Geometry: final body of the model. Coordinates: model frame, mm. A direction names the side the tool comes from. Round coordinates to 2 decimals unless told otherwise and drop trailing zeros. Order: outer loops, then holes, each group sorted by start corner. A loop starts at its lowest first (then second) coordinate and runs counter-clockwise, first axis right, second up. Notation, with made-up numbers: M -35.5,-17.5 L -30.5,-17.5 A9 ccw -30.5,-5.5 Z; hole C 47.5,59 d8. An arc over 180 degrees is marked long. Return JSON: item names as keys, results as strings. Group by question number.
Q1. Contact query for flat-ended pins moving along their axis: pin 1 (7.5 mm diameter, centred on y = -45.5, z = 6, fed in from -X); pin 2 (3.5 mm diameter, centred on x = -15, z = -2, fed in from -Y). Output: stop coordinate, or through.
Q2. Cut plane B-B on y = -4. Output: boundary loops of the cut face in (x, z), and give its area (3 significant figures).
Q3. Mould query, pull axis X, two halves, no side actions, for faces 6 (the face through (0.84, -28.9, 29.99)), 7 (the face through (-14, -1, 0)), 8 (the face through (7, 0, 0)). Classes: released by +X, released by -X, zero draft, split by the parting line, or undercut.
Q4. Ray query, probe 1 along Y at (x, z) = (0, 26); probe 2 along Z at (x, y) = (0.5, -34); probe 3 along Y at (x, z) = (-5, 21.5). Return the intervals inside material, ascending.
Q5. Access query for faces 1 (the face through (-3.707, -1, 0)), 2 (the face through (-19, 0, 0)), 3 (the face through (22.612, -29, 0)), 4 (the face through (8, -4, 0)), 5 (the face through (-17, -31.849, 0)). Directions: +Z, -Z, +X, -X, +Y, -Y. A direction counts if a zero-diameter tool reaches every point of the face in a straight line with its end or side. Return the directions, or none.
Q6. Cut plane C-C on y = -46. Output: boundary loops of the cut face in (x, z), and give its area (3 significant figures).
Q7. Cut plane A-A on z = -24. Output: boundary loops of the cut face in (x, y).
Q8. Cut plane D-D on z = -1.5. Output: boundary loops of the cut face in (x, y), and give its area (3 significant figures).
```python
from build123d import *

# Parameters (mm, degrees)
F0_R           = 30
F1_DEPTH       = 65
F3_DEPTH       = 100
F5_DEPTH       = 30.001
F6_DEPTH       = 30.001
F7_W           = 15.4366167262
F7_H           = 36.5562289953
F8_DEPTH       = 30.001
F9_DEPTH       = 30.001
F10_SIZE       = 2
F11_R          = 0.8
F12_R          = 3
F13_DEPTH      = 30.0010001
F13_DEPTH_BACK = 40
F14_DEPTH      = 8
F15_DEPTH      = 8
F16_DEPTH      = 8


with BuildPart() as f1:
    # F0 (on Front) → F1 (new body)
    with BuildSketch(Plane.XZ):
        Circle(F0_R)
    extrude(amount=F1_DEPTH)

    # F2 (on face) → F3 (cut)
    with BuildSketch(Plane.XZ.offset(65)):
        Polygon((-21.9606160964, -36.838453263), (-21.9606160964, 0), (-21.9606160964, 35.5276139707), (-38.4832583368, 35.5276139707), (-38.4832583368, -36.838453263), align=None)
        Polygon((48.3217574656, 35.5276139707), (22.611644119, 35.5276139707), (22.611644119, -36.6470105946), (22.611644119, -36.838453263), (48.3217574656, -36.838453263), align=None)
    extrude(amount=-F3_DEPTH, mode=Mode.SUBTRACT)

    # F4 (on Top) → F5 (cut, through all)
    with BuildSketch(Plane.XY):
        Polygon((-3.7071546579, 1.4132426067), (-3.7071546579, 0), (-3.7071546579, -2.5668929264), (-8, -2.5668929264), (-8, -6.3375936387), (8, -6.3375936387), (8, -2.5668929264), (2.3758972687, -2.5668929264), (2.3758972687, 0), (2.3758972687, 1.4132426067), align=None)
    extrude(amount=F5_DEPTH, mode=Mode.SUBTRACT)

    # F4 (on Top) → F6 (cut, through all)
    with BuildSketch(Plane.XY):
        Polygon((-3.7071546579, 1.4132426067), (-3.7071546579, 0), (-3.7071546579, -2.5668929264), (-8, -2.5668929264), (-8, -6.3375936387), (8, -6.3375936387), (8, -2.5668929264), (2.3758972687, -2.5668929264), (2.3758972687, 0), (2.3758972687, 1.4132426067), align=None)
    extrude(amount=-F6_DEPTH, mode=Mode.SUBTRACT)

    # F7 (on Top) → F8 (cut, through all)
    with BuildSketch(Plane.XY):
        with Locations((-20.028361585, -50.1266494393)):
            Rectangle(F7_W, F7_H)
    extrude(amount=-F8_DEPTH, mode=Mode.SUBTRACT)

    # F7 (on Top) → F9 (cut, through all)
    with BuildSketch(Plane.XY):
        with Locations((-20.028361585, -50.1266494393)):
            Rectangle(F7_W, F7_H)
    extrude(amount=F9_DEPTH, mode=Mode.SUBTRACT)

    # F10
    f10_edges = [f1.edges().sort_by_distance(p)[0] for p in [
        (-21.960616, -31.848535, 0),
    ]]
    chamfer(f10_edges, length=F10_SIZE)

    # F11
    f11_edges = [f1.edges().sort_by_distance(p)[0] for p in [
        (-12.310053, -31.848535, 0),
    ]]
    fillet(f11_edges, radius=F11_R)

    # F12 (on Top) → F13 (cut, two sides)
    with BuildSketch(Plane.XY) as f13_sk:
        with Locations((-14, 2)):
            Circle(F12_R)
        with Locations((14, 2)):
            Circle(F12_R)
    extrude(amount=F13_DEPTH, mode=Mode.SUBTRACT)
    extrude(f13_sk.sketch, amount=-F13_DEPTH_BACK, mode=Mode.SUBTRACT)

    # F14 (add): a face of the model
    f14_faces = [f1.faces().sort_by_distance(p)[0] for p in [
        (4.422443075, -65, 0),
    ]]
    extrude(f14_faces, amount=-F14_DEPTH)

    # F15 (add): a face of the model
    f15_faces = [f1.faces().sort_by_distance(p)[0] for p in [
        (4.422443075, -65, 0),
    ]]
    extrude(f15_faces, amount=-F15_DEPTH)

    # F16 (cut): a face of the model
    f16_faces = [f1.faces().sort_by_distance(p)[0] for p in [
        (4.422443075, -65, 0),
    ]]
    extrude(f16_faces, amount=-F16_DEPTH, mode=Mode.SUBTRACT)


solid = f1.part
```
Result sheet:
{
 "1": {"pin 1": "stops at x = -12.31", "pin 2": "stops at y = -31.85"},
 "2": {"outline": "M -21.96,-20.44 A30 ccw -8,-28.91 L -8,28.91 A30 ccw -21.96,20.44 Z; M 8,-28.91 A30 ccw 22.61,-19.72 L 22.61,19.72 A30 ccw 8,28.91 Z", "area": "1,450 mm²"},
 "3": {"face 6": "split by the parting line", "face 7": "undercut", "face 8": "zero draft"},
 "4": {"probe 1": "y = -57 to -6.34", "probe 2": "z = -30 to 30", "probe 3": "y = -57 to -6.34, -2.57 to 0"},
 "5": {"face 1": "+Z, -Z, +Y", "face 2": "+Z, -Z, +X, -X, +Y", "face 3": "+Z, -Z, +X, +Y, -Y", "face 4": "+Z, -Z", "face 5": "+Z, -Z, -X, -Y"},
 "6": {"outline": "M -12.31,-27.36 A30 ccw 22.61,-19.72 L 22.61,19.72 A30 ccw -12.31,27.36 Z", "area": "1,930 mm²"},
 "7": {"outline": "M -18,-31.85 L -13.11,-31.85 A0.8 cw -12.31,-32.65 L -12.31,-57 L 18,-57 L 18,0 L 16.24,0 A3 cw 11.76,0 L 2.38,0 L 2.38,-2.57 L 8,-2.57 L 8,-6.34 L -8,-6.34 L -8,-2.57 L -3.71,-2.57 L -3.71,0 L -11.76,0 A3 cw -16.24,0 L -18,0 Z"},
 "8": {"outline": "M -21.96,-29.85 L -19.96,-31.85 L -13.11,-31.85 A0.8 cw -12.31,-32.65 L -12.31,-57 L 22.61,-57 L 22.61,0 L 16.24,0 A3 cw 11.76,0 L 2.38,0 L 2.38,-2.57 L 8,-2.57 L 8,-6.34 L -8,-6.34 L -8,-2.57 L -3.71,-2.57 L -3.71,0 L -11.76,0 A3 cw -16.24,0 L -21.96,0 Z", "area": "2,210 mm²"}
}
